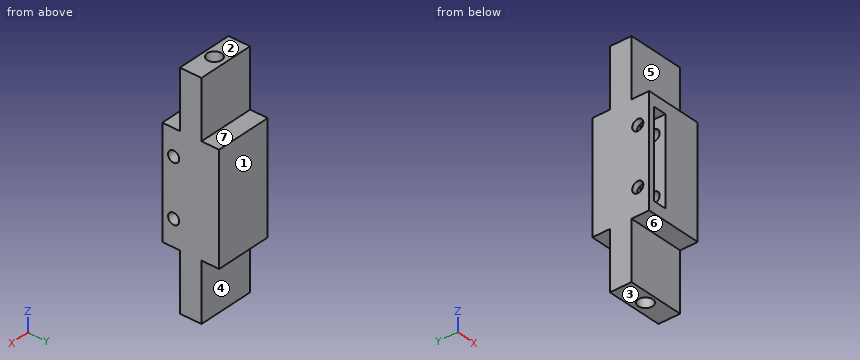
Autodesk Inventor part; units mm, degrees
ref_plane "YZ Plane" through (0, 0, 0) normal (1, 0, 0) x (0, 1, 0)
ref_plane "XZ Plane" through (0, 0, 0) normal (0, 1, 0) x (-1, 0, 0)
ref_plane "XY Plane" through (0, 0, 0) normal (0, 0, 1) x (1, 0, 0)
sketch "Sketch1" plane through (0, 0, 0) normal (0, 0, 1) x (1, 0, 0)
  line L0 (-42.4234, 22.9681) -> (-17.0234, 22.9681)
  line L1 (-17.0234, 22.9681) -> (-17.0234, -2.4319)
  line L2 (-17.0234, -2.4319) -> (-42.4234, -2.4319)
  line L3 (-42.4234, -2.4319) -> (-42.4234, 22.9681)
  point P0 (0, 0)
  dimension "d0" = 25.4
  dimension "d1" = 25.4
extrude "Extrusion1" add sketch "Sketch1" along normal blind 48.768
sketch "Sketch2" plane through (-17.0234, -2.4319, 0) normal (1, 0, 0) x (0, 0, -1)
  line L0 (-48.768, 17.526) -> (-48.768, 7.874)
  line L1 (-48.768, 7.874) -> (-74.676, 7.874)
  line L2 (-74.676, 7.874) -> (-74.676, 17.526)
  line L3 (-74.676, 17.526) -> (-48.768, 17.526)
  line L4 (-48.768, 0) -> (-48.768, 25.4)
  line L5 (0, 0) -> (-48.768, 0)
  line L6 (0, 25.4) -> (-48.768, 25.4)
  point P0 (0, 2.4319)
  dimension "d4" = 25.908
  dimension "d94" = 7.874
  dimension "d95" = 7.874
extrude "Extrusion2" add sketch "Sketch2" against normal blind 25.4
sketch "Sketch3" plane through (-17.0234, -2.4319, 0) normal (1, 0, 0) x (0, 0, -1)
  line L0 (0, 17.526) -> (0, 7.874)
  line L1 (0, 7.874) -> (25.908, 7.874)
  line L2 (25.908, 7.874) -> (25.908, 17.526)
  line L3 (25.908, 17.526) -> (0, 17.526)
  line L4 (-74.676, 7.874) -> (-48.768, 7.874)
  line L5 (-48.768, 17.526) -> (-74.676, 17.526)
  line L6 (0, 25.4) -> (0, 0)
  line L7 (0, 0) -> (-48.768, 0)
  line L8 (0, 25.4) -> (-48.768, 25.4)
  point P0 (0, 2.4319)
  point P1 (0, 22.86)
  point P2 (-55.88, 7.62)
  point P3 (-55.88, 17.78)
  point P4 (-48.768, 7.874)
  dimension "d20" = 9.652
  dimension "d23" = 9.652
  dimension "d92" = 7.874
  dimension "d96" = 25.908
  dimension "d97" = 7.874
extrude "Extrusion3" add sketch "Sketch3" against normal blind 25.4
sketch "Sketch4" plane through (-17.0234, 5.4421, 74.676) normal (0, 0, 1) x (1, 0, 0)
  line L0 (0, 9.652) -> (-25.4, 9.652)
  line L1 (-25.4, 0) -> (-25.4, 9.652)
  point P0 (17.0234, -5.4421)
  point P1 (-12.7, 4.572)
  dimension "d26" = 5.08
  dimension "d27" = 12.7
hole "Hole1" at (-29.7234, 10.0141, 74.676) direction (0, 0, -1) diameter 6.477 end through all
sketch "Sketch5" plane through (-17.0234, 22.9681, 48.768) normal (1, 0, 0) x (0, 0, -1)
  line L0 (48.768, -25.4) -> (0, -25.4)
  point P0 (48.768, -22.9681)
  point P1 (11.684, -20.32)
  point P2 (37.084, -20.32)
  dimension "d35" = 5.08
  dimension "d36" = 5.08
  dimension "d37" = 11.684
  dimension "d38" = 11.684
  dimension "d93" = 25.4
hole "Hole2" at (-17.0234, 2.6481, 37.084) at (-17.0234, 2.6481, 11.684) direction (-1, 0, 0) diameter 4.9784 end through all
sketch "Sketch19" plane through (-42.4234, -2.4319, 0) normal (0, -1, 0) x (1, 0, 0)
  line L0 (8.54, 43.688) -> (2.54, 43.688)
  line L1 (2.54, 43.688) -> (2.54, 5.08)
  line L2 (2.54, 5.08) -> (8.54, 5.08)
  line L3 (8.54, 5.08) -> (8.54, 43.688)
  line L4 (25.4, 0) -> (0, 0)
  line L5 (0, 48.768) -> (25.4, 48.768)
  line L6 (0, 0) -> (0, 48.768)
  point P0 (42.4234, 0)
  dimension "d98" = 6
  dimension "d99" = 5.08
  dimension "d100" = 5.08
  dimension "d101" = 2.54
extrude "Extrusion13" cut sketch "Sketch19" against normal blind 11.213
properties part number "SliderSlide2r"
Read the model definition and answer for the solid it produces. Units are mm, in the model's axes. Face numbers are marked on the shaded views. A direction names the side the tool comes from. Coordinates: 2 decimals unless noted, no trailing zeros. Order: outer loops, then holes, each group sorted by start corner. A loop starts at its lowest first (then second) coordinate and runs counter-clockwise, first axis right, second up. Notation, with made-up numbers: (-9, 89.5) - (47, 89.5) arc R25 ccw to (47, 106.5) - close; hole circle Ø1 at (47.5, 26). An arc over 180 degrees is marked (long way). Answer as a JSON object with one key per item and string values. Group by question number.
Item 1: Section D-D (y = 21.25) is taken. Give the vertices of the cut face in (x, z), plus the area to 3 significant figures.
Item 2: Section C-C (z = 42) is taken. Give the vertices of the cut face in (x, y).
Item 3: Consider probe 1 along Z at (x, y) = (-39.5, 6.25); probe 2 along X at (y, z) = (4.25, 18); probe 3 along Z at (x, y) = (-23, 2). Determine where each line is inside the solid, lowest interval first. Write a range as from..to.
Item 4: The mould has two halves that part along Z. Classify the marked faces 1, 2 and 3: +Z half, -Z half, draft (parallel to the pull), parting line (faces both ways), or undercut.
Item 5: Section A-A (x = -28.5) is taken. Give the vertices of the cut face in (y, z).
Item 6: A tool of negligible diameter and unlimited length cuts with its end or side. For the marked faces 4, 5, 6 and 7, from which of +Z, -Z, +X, -X, +Y, -Y can it reach the whole face along a straight path? Write none if from no direction.
Item 7: Section B-B (y = 10.5) is taken. Give the vertices of the cut face in (x, z), plus the area to 3 significant figures.
Item 8: Flat-ended cylindrical pins translate along their axes: P1, Ø2.5, axis at x = -33.5, y = 17.5, coming from the -Z side; P2, Ø2.5, axis at x = -24, y = 0.5, coming from the +Z side; P3, Ø7.5, axis at x = -33, z = -15, coming from the -Y side; P4, Ø6.5, axis at y = 2.65, z = 11.68, coming from the -X side. Find the tip coordinate at first contact, or state that the pin passes through.
Results are:
{
 "1": {"outline": "(-42.42, 0) - (-17.02, 0) - (-17.02, 48.77) - (-42.42, 48.77) - close", "area": "1,240 mm^2"},
 "2": {"outline": "(-42.42, -2.43) - (-39.88, -2.43) - (-39.88, 8.78) - (-33.88, 8.78) - (-33.88, -2.43) - (-17.02, -2.43) - (-17.02, 22.97) - (-42.42, 22.97) - close; hole circle Ø6.48 at (-29.72, 10.01)"},
 "3": {"probe 1": "z = -25.91..5.08, 43.69..74.68", "probe 2": "x = -42.42..-39.88, -33.88..-17.02", "probe 3": "z = 0..9.28, 14.09..34.68, 39.49..48.77"},
 "4": {"face 1": "draft", "face 2": "+Z half", "face 3": "-Z half"},
 "5": {"outline": "(-2.43, 0) - (5.44, 0) - (5.44, -25.91) - (7.02, -25.91) - (7.02, 74.68) - (5.44, 74.68) - (5.44, 48.77) - (-2.43, 48.77) - close; (13.01, -25.91) - (15.09, -25.91) - (15.09, 0) - (22.97, 0) - (22.97, 48.77) - (15.09, 48.77) - (15.09, 74.68) - (13.01, 74.68) - close; hole circle Ø4.98 at (2.65, 11.68); hole circle Ø4.98 at (2.65, 37.08)"},
 "6": {"face 4": "-Z, +X, -X, +Y", "face 5": "+Z, +X, -X, -Y", "face 6": "-Z, +X, -X, -Y", "face 7": "+Z, +X, -X, +Y"},
 "7": {"outline": "(-42.42, -25.91) - (-32.93, -25.91) - (-32.93, 74.68) - (-42.42, 74.68) - close; (-26.52, -25.91) - (-17.02, -25.91) - (-17.02, 74.68) - (-26.52, 74.68) - close", "area": "1,910 mm^2"},
 "8": {"P1": "stops at z = 0", "P2": "stops at z = 48.77", "P3": "stops at y = 5.44", "P4": "stops at x = -42.42"}
}
